Can you work these out from the drawing? Everything is in mm from the part's minimum corner. A direction names the side the tool comes from. Give positions to 0.01 mm unless a question says otherwise; leave off trailing zeros. Write each loop counter-clockwise with the first axis right and the second up, starting at its lowest first coordinate (ties: lowest second). Pieces come first, ordered by that corner, then holes. Notation, with made-up numbers: M 56,83 L 106,83 A16 cw 106,111 Z; hole C 34,39 d3. An arc over 180 degrees is marked long. One line per item, written item: value.
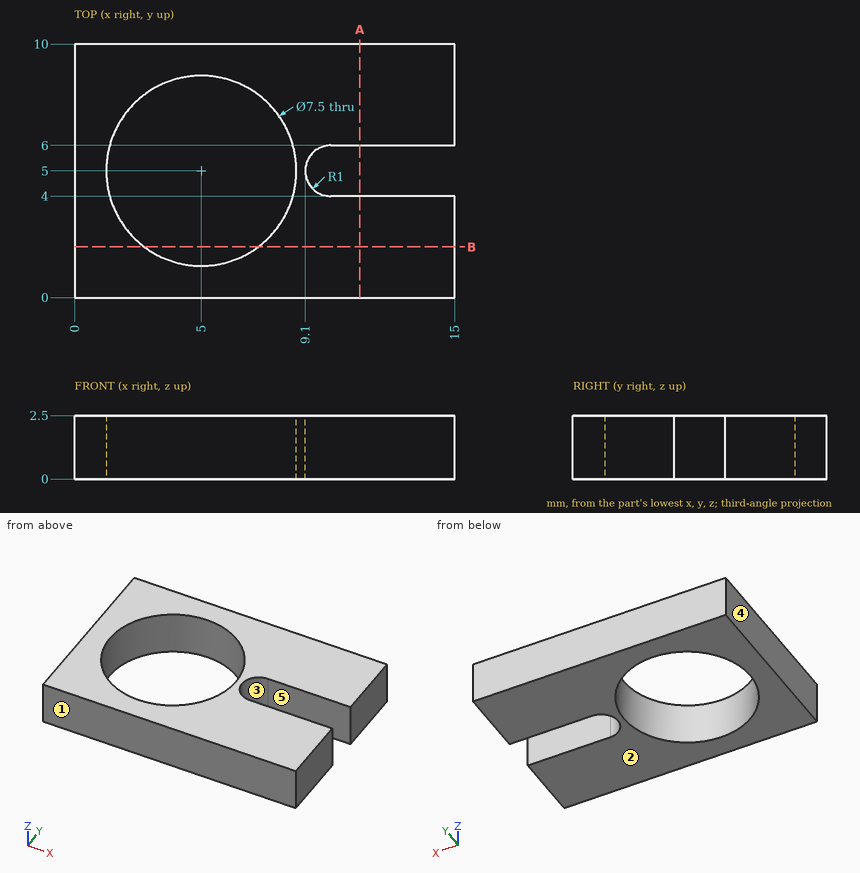
1) We'd pull the mould along Y, two halves only. Please class the marked faces 1, 2 and 3: pulls with the +Y half, pulls with the -Y half, needs draft (parallel to the pull), parting line crosses it, or undercut.
Outcome:
face 1: pulls with the -Y half
face 2: needs draft
face 3: undercut
2) On a 3-axis mill with a long thin cutter (end or side, diameter ignored), from which of +Z, -Z, +X, -X, +Y, -Y can I reach the whole of each face in a straight line? I mean the marked faces 4 and 5. Say none if no direction works.
Outcome:
face 4: +Z, -Z, -X, +Y, -Y
face 5: +Z, -Z, +X
3) Please list where these lines run through material, in increasing order: L1, parallel to Y at x = 5, z = 1.5; L2, parallel to Y at x = 10.5, z = 1.45; L3, parallel to X at y = 8, z = 1.1. Write a range as from..to.
Outcome:
L1: y = 0..1.25, 8.75..10
L2: y = 0..4, 6..10
L3: x = 0..2.75, 7.25..15
4) If we section it at A-A, the plane x = 11.25: Write out the boundary of the cut face in (y, z).
Outcome:
outline: M 0,0 L 4,0 L 4,2.5 L 0,2.5 Z; M 6,0 L 10,0 L 10,2.5 L 6,2.5 Z
5) If we section it at B-B, the plane y = 2: Write out the boundary of the cut face in (x, z).
Outcome:
outline: M 0,0 L 2.75,0 L 2.75,2.5 L 0,2.5 Z; M 7.25,0 L 15,0 L 15,2.5 L 7.25,2.5 Z
